Check sheet for the modelled part. Datum: model origin and axes. Units: mm. Round coordinates to 2 decimals unless told otherwise and drop trailing zeros. Order: outer loops, then holes, each group sorted by start corner. A loop starts at its lowest first (then second) coordinate and runs counter-clockwise, first axis right, second up. Notation, with made-up numbers: (-30, -24) -> (1, -24) arc R24 ccw to (1, 11) -> close; hole circle Ø9 at (1.5, 47.25). An arc over 180 degrees is marked (long way). Answer in a Markdown table with one row per item.
Autodesk Inventor part; units mm, degrees
ref_plane "YZ Plane" through (0, 0, 0) normal (1, 0, 0) x (0, 1, 0)
ref_plane "XZ Plane" through (0, 0, 0) normal (0, 1, 0) x (-1, 0, 0)
ref_plane "XY Plane" through (0, 0, 0) normal (0, 0, 1) x (1, 0, 0)
sketch "Sketch1" plane through (0, 0, 0) normal (0, 0, 1) x (1, 0, 0)
  line L0 (0, 0) -> (38.1, 0)
  line L1 (38.1, 0) -> (38.1, 25.4)
  line L2 (38.1, 25.4) -> (0, 25.4)
  line L3 (0, 25.4) -> (0, 0)
  circle A0 centre (6.35, 12.7) radius 2.0701
  circle A1 centre (31.75, 12.7) radius 2.0701
  dimension "d0" = 38.1
  dimension "d1" = 25.4
  dimension "d2" = 4.1402
  dimension "d3" = 6.35
  dimension "d4" = 12.7
  dimension "d24" = 25.4
extrude "Extrusion1" add sketch "Sketch1" along normal blind 3.175
fillet "Fillet1" radius 3.175 4 edges at (38.1, 25.4, 1.5875) (38.1, 0, 1.5875) (0, 25.4, 1.5875) (0, 0, 1.5875)
properties part number "Spacer 2" material "Aluminum 6061"
Item 1: Mould release check, pull along Y, two halves, no side actions. Record for faces 1 (the cylindrical face through (29.68, 12.61, 1.57)), 2 (the flat face through (38.1, 13, 2)), 3 (the flat face through (19, 0, 2)): pulls with the +Y half, pulls with the -Y half, needs draft (parallel to the pull), parting line crosses it, or undercut.
Result sheet:
| item | result |
|---|---|
| face 1 | undercut |
| face 2 | needs draft |
| face 3 | pulls with the -Y half |
Item 2: Scan lines: line 1 (X direction, y = 12.75, z = 2.6); line 2 (Y direction, x = 31.75, z = 2.45); line 3 (X direction, y = 11.25, z = 3). Record each from-to range of solid material in increasing order. Write a range as [from, to].
Result sheet:
| item | result |
|---|---|
| line 1 | x = [0, 4.28], [8.42, 29.68], [33.82, 38.1] |
| line 2 | y = [0, 10.63], [14.77, 25.4] |
| line 3 | x = [0, 4.87], [7.83, 30.27], [33.23, 38.1] |
Item 3: Cross-section at C-C (z = 1.65). Record the boundary of the cut face in (x, y) (3 decimals).
Result sheet:
| item | result |
|---|---|
| outline | (0, 3.175) arc R3.175 ccw to (3.175, 0) -> (34.925, 0) arc R3.175 ccw to (38.1, 3.175) -> (38.1, 22.225) arc R3.175 ccw to (34.925, 25.4) -> (3.175, 25.4) arc R3.175 ccw to (0, 22.225) -> close; hole circle Ø4.14 at (6.35, 12.7); hole circle Ø4.14 at (31.75, 12.7) |
Item 4: Cross-section at D-D (x = 31.5). Record the boundary of the cut face in (y, z) (3 decimals).
Result sheet:
| item | result |
|---|---|
| outline | (0, 0) -> (10.645, 0) -> (10.645, 3.175) -> (0, 3.175) -> close; (14.755, 0) -> (25.4, 0) -> (25.4, 3.175) -> (14.755, 3.175) -> close |
Item 5: Cross-section at B-B (y = 12.7). Record the boundary of the cut face in (x, z) (3 decimals).
Result sheet:
| item | result |
|---|---|
| outline | (0, 0) -> (4.28, 0) -> (4.28, 3.175) -> (0, 3.175) -> close; (8.42, 0) -> (29.68, 0) -> (29.68, 3.175) -> (8.42, 3.175) -> close; (33.82, 0) -> (38.1, 0) -> (38.1, 3.175) -> (33.82, 3.175) -> close |
Item 6: Cross-section at A-A (x = 6.35). Record the boundary of the cut face in (y, z) (3 decimals), and give its area (3 significant figures).
Result sheet:
| item | result |
|---|---|
| outline | (0, 0) -> (10.63, 0) -> (10.63, 3.175) -> (0, 3.175) -> close; (14.77, 0) -> (25.4, 0) -> (25.4, 3.175) -> (14.77, 3.175) -> close |
| area | 67.5 mm^2 |
